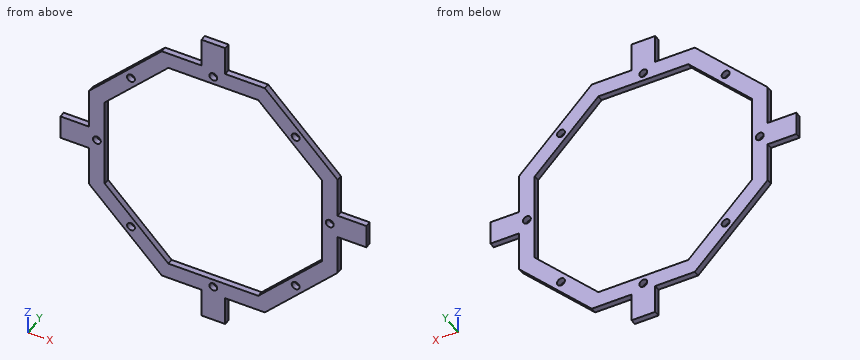
```python
from build123d import *

# Parameters (mm, degrees)
BOSS_EXTRUDE1_DEPTH     = 3
CUT_EXTRUDE1_DEPTH      = 84
CUT_EXTRUDE1_DEPTH_BACK = 76
SKETCH3_R               = 2


with BuildPart() as part:
    # Sketch2 → Boss-Extrude1 (new body)
    with BuildSketch(Plane(origin=(0, 0, 0), x_dir=(1, 0, 0), z_dir=(0, 1, 0))):
        Polygon((6, -77.5), (6, -63), (26.09545443, -63), (63, -26.09545443), (63, -6), (77.5, -6), (77.5, 6), (63, 6), (63, 26.09545443), (26.09545443, 63), (6, 63), (6, 77.5), (-6, 77.5), (-6, 63), (-26.09545443, 63), (-63, 26.09545443), (-63, 6), (-77.5, 6), (-77.5, -6), (-63, -6), (-63, -26.09545443), (-26.09545443, -63), (-6, -63), (-6, -77.5), align=None)
        Polygon((22.781745931, -55), (55, -22.781745931), (55, 22.781745931), (22.781745931, 55), (-22.781745931, 55), (-55, 22.781745931), (-55, -22.781745931), (-22.781745931, -55), align=None, mode=Mode.SUBTRACT)
    extrude(amount=BOSS_EXTRUDE1_DEPTH)

    # Sketch3 → Cut-Extrude1 (cut, two sides: drawn at the far end of the back side and taken through both)
    with BuildSketch(Plane(origin=(0, 3, 0), x_dir=(1, 0, 0), z_dir=(0, 1, 0)).offset(-CUT_EXTRUDE1_DEPTH_BACK)):
        with Locations(Location((0, 59, 0), (0, 0, 270))):
            Circle(SKETCH3_R)
        with Locations(Location((41.71930009, 41.71930009, 0), (0, 0, 270))):
            Circle(SKETCH3_R)
        with Locations(Location((59, 0, 0), (0, 0, 270))):
            Circle(SKETCH3_R)
        with Locations(Location((41.71930009, -41.71930009, 0), (0, 0, 270))):
            Circle(SKETCH3_R)
        with Locations(Location((0, -59, 0), (0, 0, 270))):
            Circle(SKETCH3_R)
        with Locations(Location((-41.71930009, -41.71930009, 0), (0, 0, 270))):
            Circle(SKETCH3_R)
        with Locations(Location((-59, 0, 0), (0, 0, 270))):
            Circle(SKETCH3_R)
        with Locations(Location((-41.71930009, 41.71930009, 0), (0, 0, 270))):
            Circle(SKETCH3_R)
    extrude(amount=CUT_EXTRUDE1_DEPTH + CUT_EXTRUDE1_DEPTH_BACK, mode=Mode.SUBTRACT)


solid = part.part
```
Design review of the part built by this model. Coordinates are the model's own, in mm. Round coordinates to 2 decimals unless told otherwise and drop trailing zeros. Write each loop counter-clockwise with the first axis right and the second up, starting at its lowest first coordinate (ties: lowest second). Pieces come first, ordered by that corner, then holes. Notation, with made-up numbers: (78, -2.75) -> (121, -2.75) arc R12 ccw to (121, 2.25) -> close; hole circle Ø2 at (3, 10.25). An arc over 180 degrees is marked (long way). Answer in a Markdown table with one row per item.
Q1. Take a section at A-A, the plane z = -17. State the section outline as (x, y) points.
The answers:
| item | result |
|---|---|
| outline | (-63, 0) -> (-55, 0) -> (-55, 3) -> (-63, 3) -> close; (55, 0) -> (63, 0) -> (63, 3) -> (55, 3) -> close |
Q2. Take a section at C-C, the plane z = 0. State the section outline as (x, y) points.
The answers:
| item | result |
|---|---|
| outline | (-77.5, 0) -> (-61, 0) -> (-61, 3) -> (-77.5, 3) -> close; (-57, 0) -> (-55, 0) -> (-55, 3) -> (-57, 3) -> close; (55, 0) -> (57, 0) -> (57, 3) -> (55, 3) -> close; (61, 0) -> (77.5, 0) -> (77.5, 3) -> (61, 3) -> close |
Q3. Take a section at B-B, the plane x = 0. State the section outline as (y, z) points, then the cut area to 3 significant figures.
The answers:
| item | result |
|---|---|
| outline | (0, -77.5) -> (3, -77.5) -> (3, -61) -> (0, -61) -> close; (0, -57) -> (3, -57) -> (3, -55) -> (0, -55) -> close; (0, 55) -> (3, 55) -> (3, 57) -> (0, 57) -> close; (0, 61) -> (3, 61) -> (3, 77.5) -> (0, 77.5) -> close |
| area | 111 mm² |
Q4. To check wall thickness, follow L1, parallel to X at y = 1.45, z = 0; L2, parallel to X at y = 2.35, z = -19; L3, parallel to Z at x = -66.5, y = 2.35. State the ranges of each line that lie inside material, in increasing order. Write a range as [from, to].
The answers:
| item | result |
|---|---|
| L1 | [-77.5, -61], [-57, -55], [55, 57], [61, 77.5] |
| L2 | [-63, -55], [55, 63] |
| L3 | [-6, 6] |
Q5. Take a section at D-D, the plane x = -30. State the section outline as (y, z) points.
The answers:
| item | result |
|---|---|
| outline | (0, -59.1) -> (3, -59.1) -> (3, -47.78) -> (0, -47.78) -> close; (0, 47.78) -> (3, 47.78) -> (3, 59.1) -> (0, 59.1) -> close |
Q6. Clearance check with flat-ended pins moving along their axes: pin 1 Ø1.5 at (x, y) = (-68.5, 2) entering from -Z; pin 2 Ø0.9 at (y, z) = (1, 73) entering from -X; pin 3 Ø1.5 at (y, z) = (2, -18.5) entering from +X. State where each tip first meets the part, or that it passes through.
The answers:
| item | result |
|---|---|
| pin 1 | z = -6 |
| pin 2 | x = -6 |
| pin 3 | x = 63 |
